Geometry: see drawing. Coordinates: mm, zero at the bounding-box minimum. Coordinates: 2 decimals unless noted, no trailing zeros. Write each loop counter-clockwise with the first axis right and the second up, starting at its lowest first coordinate (ties: lowest second). Pieces come first, ordered by that corner, then holes. Notation, with made-up numbers: (70.25, 53.5) -> (87.25, 53.5) arc R13 cw to (87.25, 65.5) -> close; hole circle Ø11 at (83.5, -34.75). An arc over 180 degrees is marked (long way). Use one line per item in the form item = value. Start each with the question number.
(1) First-contact query: pin 1 (2 mm diameter, centred on x = 21, y = 38, fed in from -Z). Flat tip, straight axial feed; report the tip coordinate or a pass-through.
(2) Cut plane B-B on z = 18.5. Return the cut outline in (x, y), plus the area to 3 significant figures.
(3) Pull-direction query (X, two-part tool) for the marked faces 1, 2, 3 and 4; classes: released by +X, released by -X, zero draft, split by the parting line, or undercut.
(4) Cut plane A-A on z = 2.25. Return the cut outline in (x, y), plus the area to 3 significant figures.
(5) Ray query, line 1 along Y through (x, z) = (24, 7.75); line 2 along X through (y, z) = (36, 17.5) (1 decimal); line 3 along Y through (x, z) = (26, 6.75) (1 decimal). Return the intervals inside material, ascending.
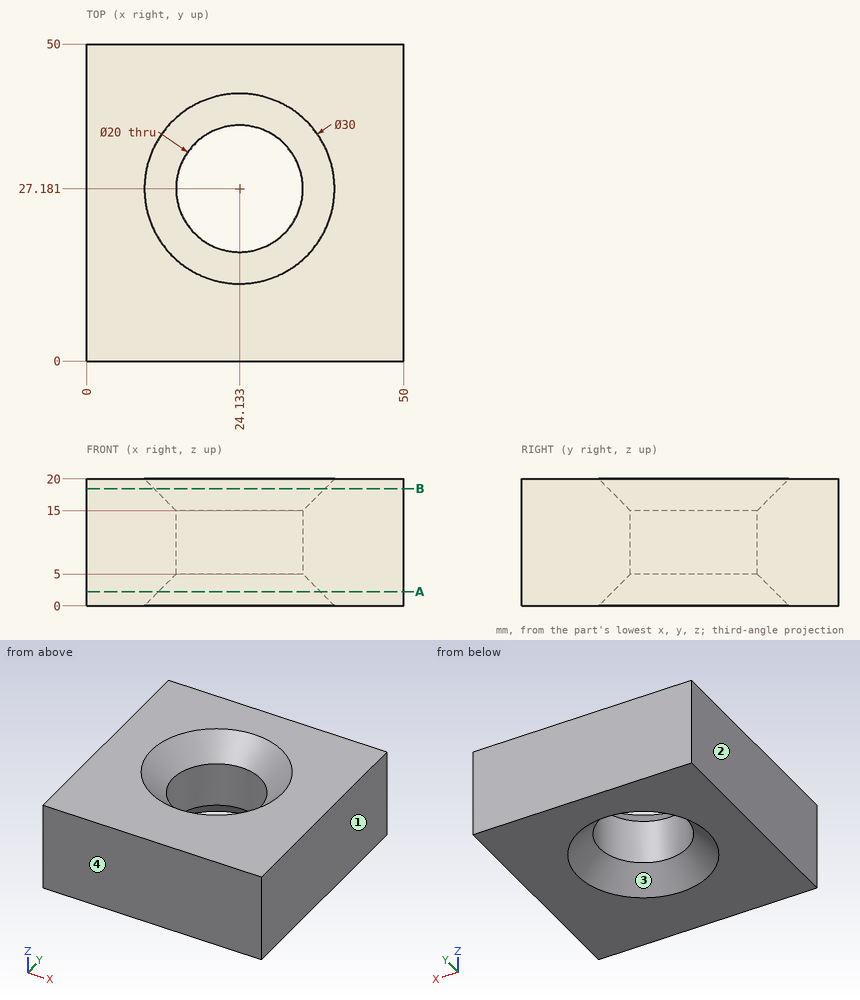
Values:
q1.pin_1 = 2.74
q2.outline = (0, 0) -> (50, 0) -> (50, 50) -> (0, 50) -> close; hole circle Ø27 at (24.13, 27.18)
q2.area = 1,930 mm2
q3.face_1 = released by +X
q3.face_2 = released by -X
q3.face_3 = undercut
q3.face_4 = zero draft
q4.outline = (0, 0) -> (50, 0) -> (50, 50) -> (0, 50) -> close; hole circle Ø25.5 at (24.13, 27.18)
q4.area = 1,990 mm2
q5.line_1 = 0 to 17.18, 37.18 to 50
q5.line_2 = 0 to 15.3, 33 to 50
q5.line_3 = 0 to 17.4, 37 to 50
